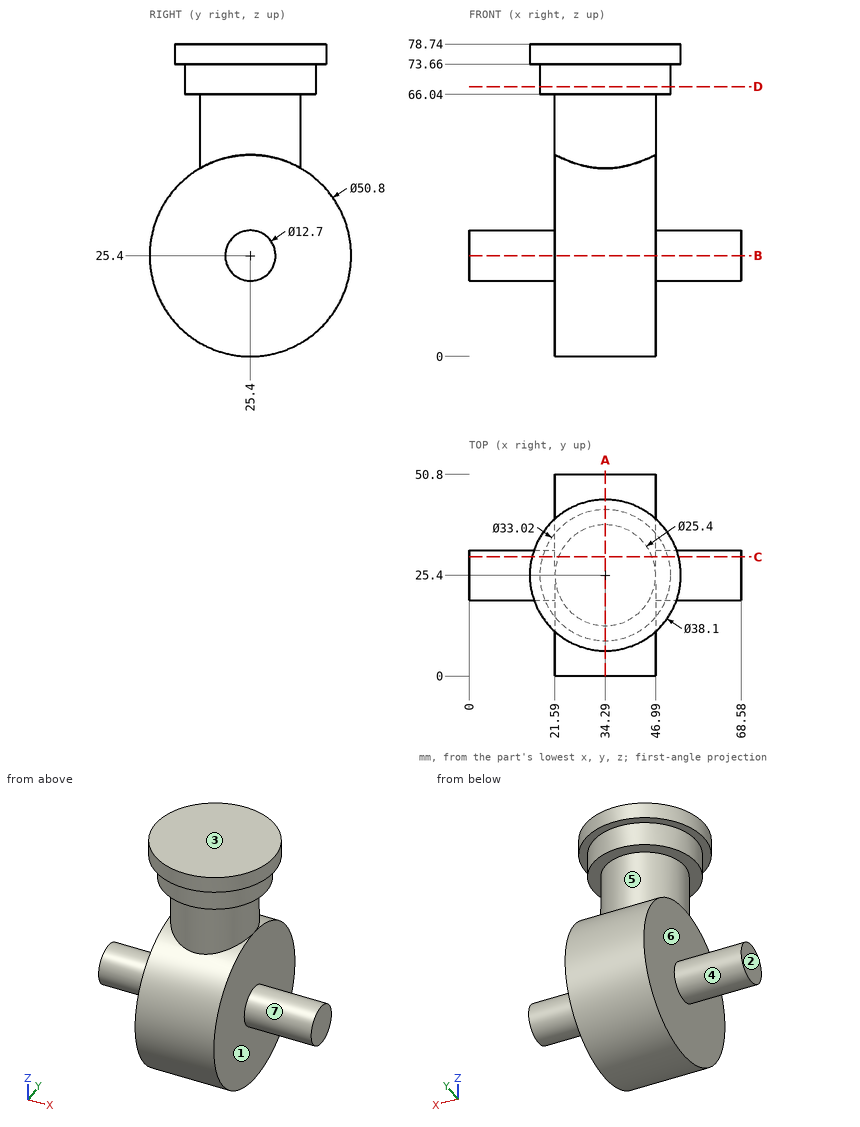
Geometry: see drawing. Coordinates: mm, zero at the bounding-box minimum. A direction names the side the tool comes from. Give positions to 0.01 mm unless a question says otherwise; leave off trailing zeros. Write each loop counter-clockwise with the first axis right and the second up, starting at its lowest first coordinate (ties: lowest second). Pieces come first, ordered by that corner, then holes. Notation, with made-up numbers: M 61,71.5 L 86,71.5 A13 ccw 86,95.5 Z; hole C 73,-1 d11. An arc over 180 degrees is marked long. Answer as a JSON object with one key per item and string values.
Q1. Cut plane C-C, the plane y = 30. Return the cut outline in (x, z), then the cut area to 3 significant figures.
Geometry check:
{"outline": "M 0,21.02 L 21.59,21.02 L 21.59,0.42 L 46.99,0.42 L 46.99,21.02 L 68.58,21.02 L 68.58,29.78 L 46.99,29.78 L 46.99,50.38 L 46.13,50.38 L 46.13,66.04 L 50.15,66.04 L 50.15,73.66 L 52.78,73.66 L 52.78,78.74 L 15.8,78.74 L 15.8,73.66 L 18.43,73.66 L 18.43,66.04 L 22.45,66.04 L 22.45,50.38 L 21.59,50.38 L 21.59,29.78 L 0,29.78 Z", "area": "2,450 mm^2"}
Q2. Cut plane B-B, the plane z = 25.4. Return the cut outline in (x, y), then the cut area to 3 significant figures.
Geometry check:
{"outline": "M 0,19.05 L 21.59,19.05 L 21.59,0 L 46.99,0 L 46.99,19.05 L 68.58,19.05 L 68.58,31.75 L 46.99,31.75 L 46.99,50.8 L 21.59,50.8 L 21.59,31.75 L 0,31.75 Z", "area": "1,840 mm^2"}
Q3. Ray query, line 1 along Z through (x, y) = (23.5, 25); line 2 along X through (y, z) = (22.5, 16); line 3 along Z through (x, y) = (17.5, 25.5). Return the intervals inside material, ascending.
Geometry check:
{"line 1": "z = 0 to 78.74", "line 2": "x = 21.59 to 46.99", "line 3": "z = 19.05 to 31.75, 73.66 to 78.74"}
Q4. Contact query for flat-ended pins moving along their axis: P1, Ø5, axis at y = 39, z = 64, coming from the -X side; P2, Ø11.5, axis at x = 40.5, y = 16.5, coming from the -Z side; P3, Ø1, axis at y = 29.5, z = 41.5, coming from the +X side. Output: stop coordinate, or through.
Geometry check:
{"P1": "stops at x = 23.12", "P2": "stops at z = 0.2", "P3": "stops at x = 46.99"}
Q5. Cut plane A-A, the plane x = 34.29. Return the cut outline in (y, z).
Geometry check:
{"outline": "M 6.35,73.66 L 8.89,73.66 L 8.89,66.04 L 12.7,66.04 L 12.7,47.4 A25.4 ccw long 38.1,47.4 L 38.1,66.04 L 41.91,66.04 L 41.91,73.66 L 44.45,73.66 L 44.45,78.74 L 6.35,78.74 Z"}
Q6. Mould query, pull axis Z, two halves, no side actions, for the marked faces 1, 2, 3 and 4. Classes: +Z half, -Z half, draft (parallel to the pull), parting line (faces both ways), or undercut.
Geometry check:
{"face 1": "undercut", "face 2": "draft", "face 3": "+Z half", "face 4": "undercut"}
Q7. Access query for the marked faces 5, 6 and 7. Directions: +Z, -Z, +X, -X, +Y, -Y. A direction counts if a zero-diameter tool reaches every point of the face in a straight line with its end or side. Return the directions, or none.
Geometry check:
{"face 5": "none", "face 6": "-X", "face 7": "+X"}
Q8. Cut plane D-D, the plane z = 68. Return the cut outline in (x, y), then the cut area to 3 significant figures.
Geometry check:
{"outline": "C 34.29,25.4 d33.02", "area": "856 mm^2"}
